Verification items for this drawing (mm, ordinates from the low corner). A direction names the side the tool comes from. Coordinates: 2 decimals unless noted, no trailing zeros. Loops run counter-clockwise (first coordinate to the right, second up) from the corner with the lowest first, then second, coordinate; pieces in that order, holes last. Notation, with made-up numbers: (5, 20) - (32, 20) arc R12 cw to (32, 43) - close; hole circle Ø8 at (16, -17.5). An arc over 180 degrees is marked (long way). One line per item, written item: value. Start each with the question number.
(1) Section check C-C (y = 39). Record the boundary of the cut face in (x, z).
(2) Gauge pin test, flat ends, axial feed: P1, Ø8, axis at y = 25, z = 11, coming from the +X side; P2, Ø1.5, axis at x = 30.5, z = 8.5, coming from the -Y side; P3, Ø3, axis at x = 23, y = 19.5, coming from the -Z side. Record the tip position at first contact, or that the pin passes through.
(3) Draft check along X on the marked faces 1, 2 and 3. Enter one of: +X half, -X half, draft (parallel to the pull), parting line (faces both ways), or undercut.
(4) Section check A-A (z = 8.5). Record the boundary of the cut face in (x, y).
(5) Section check D-D (y = 15.5). Record the boundary of the cut face in (x, z).
(6) Section check B-B (x = 41). Record the boundary of the cut face in (y, z), plus the area to 3 significant figures.
(7) Thickness scan on probe 1 along X at (y, z) = (41, 10.5); probe 2 along X at (y, z) = (26, 1); probe 3 along Y at (x, z) = (21, 7.75). Record the ranges inside material, lowest first. Write a range as [from, to].
(8) Set-up check for the marked faces 4, 5 and 6: record each of +Z, -Z, +X, -X, +Y, -Y from which the full face is reachable in a straight line by a thin tool's end or side.
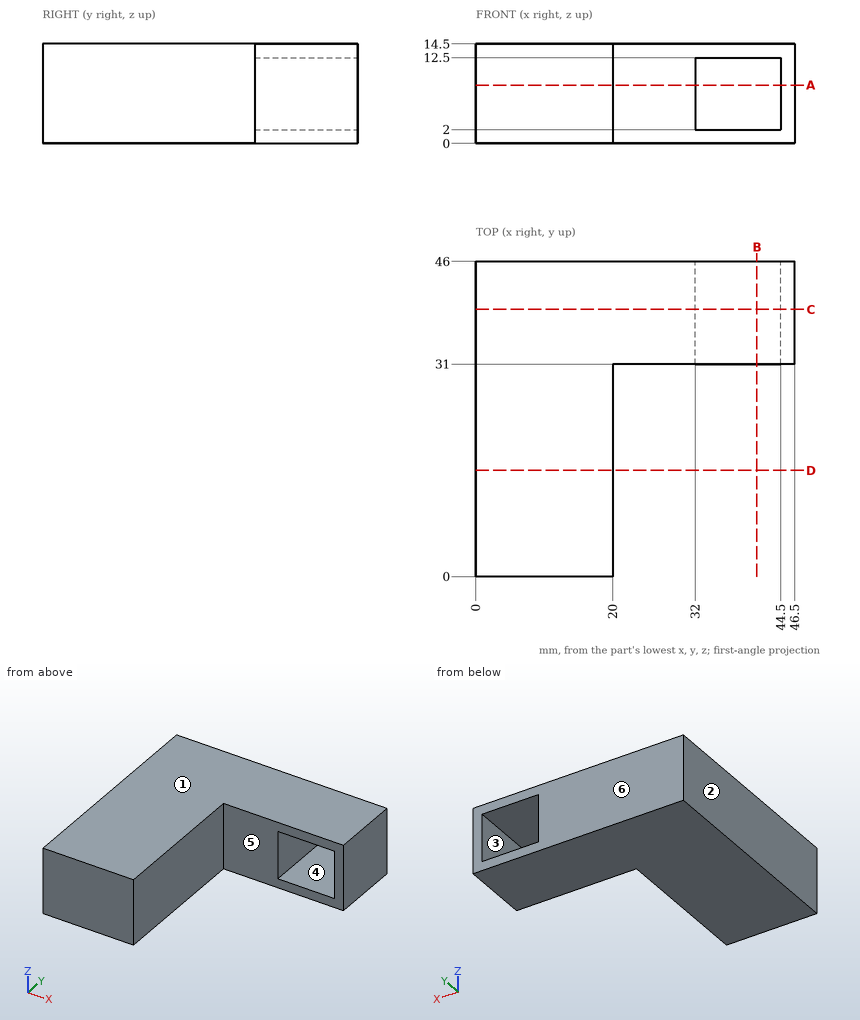
Responses:
1. outline: (0, 0) - (46.5, 0) - (46.5, 14.5) - (0, 14.5) - close; hole (32, 2) - (44.5, 2) - (44.5, 12.5) - (32, 12.5) - close
2. P1: stops at x = 20
2. P2: stops at y = 31
2. P3: passes through
3. face 1: draft
3. face 2: -X half
3. face 3: undercut
4. outline: (0, 0) - (20, 0) - (20, 31) - (32, 31) - (32, 46) - (0, 46) - close; (44.5, 31) - (46.5, 31) - (46.5, 46) - (44.5, 46) - close
5. outline: (0, 0) - (20, 0) - (20, 14.5) - (0, 14.5) - close
6. outline: (31, 0) - (46, 0) - (46, 2) - (31, 2) - close; (31, 12.5) - (46, 12.5) - (46, 14.5) - (31, 14.5) - close
6. area: 60.0 mm²
7. probe 1: x = [0, 32], [44.5, 46.5]
7. probe 2: x = [0, 20]
7. probe 3: y = [31, 46]
8. face 4: +Y, -Y
8. face 5: +Z, -Z, +X, -Y
8. face 6: +Z, -Z, +X, -X, +Y
